Part model, mm, in its own coordinate system. Coordinates: 2 decimals unless noted, no trailing zeros. Loops run counter-clockwise (first coordinate to the right, second up) from the corner with the lowest first, then second, coordinate; pieces in that order, holes last. Notation, with made-up numbers: M 24,79 L 68,79 A23 ccw 68,89 Z; hole C 66,-37.75 d8. An arc over 180 degrees is marked long. Use a Markdown table: item, result. Add a question column.
1) Band-saw the part on D-D (y = 5). List the corners of the cut face in (x, z), plus the area to 3 significant figures.
2) Band-saw the part on A-A (x = 91). List the corners of the cut face in (y, z), plus the area to 3 significant figures.
3) Wall check: probe 1 along X at (y, z) = (35, 1.2); probe 2 along Y at (x, z) = (83, 0.8); probe 3 along X at (y, z) = (117, 1.55). Give the ranges that are in metal, low to high. Write a range as from..to.
4) Band-saw the part on B-B (y = 31). List the corners of the cut face in (x, z), plus the area to 3 significant figures.
5) Band-saw the part on C-C (x = 40). List the corners of the cut face in (y, z).
6) Pin check, flat tips, straight feed: pin 1 Ø0.8 at (x, z) = (101, 2.5) entering from +Y; pin 2 Ø0.8 at (y, z) = (28.5, 2.5) entering from -X; pin 3 Ø3.5 at (x, y) = (40, 117) entering from +Z. Stop position of each tip, or through.
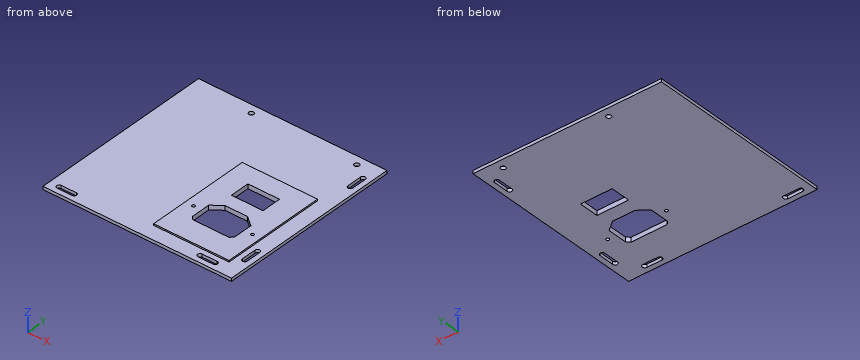
from build123d import *

# Parameters (mm, degrees)
SKETCH_W        = 125
SKETCH_H        = 123
PAD_DEPTH       = 2
SKETCH001_W     = 50
SKETCH001_H     = 70
PAD001_DEPTH    = 3
POCKET_DEPTH    = 3.001
POCKET001_DEPTH = 3.001
SKETCH004_R     = 1.6
POCKET002_DEPTH = 3.001
SKETCH005_R     = 1.6
POCKET003_DEPTH = 3.001
POCKET004_DEPTH = 3.001
SKETCH007_R     = 1
POCKET005_DEPTH = 3.001
SKETCH008_R     = 1
POCKET006_DEPTH = 3.001
SKETCH009_W     = 21
SKETCH009_H     = 13
POCKET007_DEPTH = 3.001
POCKET008_DEPTH = 3.001
POCKET009_DEPTH = 3.001


with BuildPart() as part:
    # Sketch → Pad (new body)
    with BuildSketch(Plane.XY):
        with Locations((62.5, 61.5)):
            Rectangle(SKETCH_W, SKETCH_H)
    extrude(amount=PAD_DEPTH)

    # Sketch001 → Pad001 (join)
    with BuildSketch(Plane.XY):
        with Locations((90, 45)):
            Rectangle(SKETCH001_W, SKETCH001_H)
    extrude(amount=PAD001_DEPTH)

    # Sketch002 → Pocket (cut, through all)
    with BuildSketch(Plane.XY):
        with BuildLine():
            ThreePointArc((6.55, 6.6), (4.95, 5), (6.55, 3.4))
            Line((6.55, 3.4), (16.55, 3.4))
            ThreePointArc((16.55, 3.4), (18.15, 5), (16.55, 6.6))
            Line((6.55, 6.6), (16.55, 6.6))
        make_face()
    extrude(amount=POCKET_DEPTH, mode=Mode.SUBTRACT)

    # Sketch003 → Pocket001 (cut, through all)
    with BuildSketch(Plane.XY):
        with BuildLine():
            ThreePointArc((121.6, 26.55), (120, 28.15), (118.4, 26.55))
            Line((118.4, 26.55), (118.4, 16.55))
            ThreePointArc((118.4, 16.55), (120, 14.95), (121.6, 16.55))
            Line((121.6, 26.55), (121.6, 16.55))
        make_face()
    extrude(amount=POCKET001_DEPTH, mode=Mode.SUBTRACT)

    # Sketch004 → Pocket002 (cut, through all)
    with BuildSketch(Plane.XY):
        with Locations((110, 117)):
            Circle(SKETCH004_R)
    extrude(amount=POCKET002_DEPTH, mode=Mode.SUBTRACT)

    # Sketch005 → Pocket003 (cut, through all)
    with BuildSketch(Plane.XY):
        with Locations((40, 117)):
            Circle(SKETCH005_R)
    extrude(amount=POCKET003_DEPTH, mode=Mode.SUBTRACT)

    # Sketch006 → Pocket004 (cut, through all)
    with BuildSketch(Plane.XY):
        Polygon((76, 40.43372), (82.5, 45.5), (97.5, 45.5), (104, 40.435902), (104, 27.5), (102, 25.5), (78, 25.5), (76, 27.5), align=None)
    extrude(amount=POCKET004_DEPTH, mode=Mode.SUBTRACT)

    # Sketch007 → Pocket005 (cut, through all)
    with BuildSketch(Plane.XY):
        with Locations((70.5, 35)):
            Circle(SKETCH007_R)
    extrude(amount=POCKET005_DEPTH, mode=Mode.SUBTRACT)

    # Sketch008 → Pocket006 (cut, through all)
    with BuildSketch(Plane.XY):
        with Locations((109.5, 35)):
            Circle(SKETCH008_R)
    extrude(amount=POCKET006_DEPTH, mode=Mode.SUBTRACT)

    # Sketch009 → Pocket007 (cut, through all)
    with BuildSketch(Plane.XY):
        with Locations((89.75, 61)):
            Rectangle(SKETCH009_W, SKETCH009_H)
    extrude(amount=POCKET007_DEPTH, mode=Mode.SUBTRACT)

    # Sketch010 → Pocket008 (cut, through all)
    with BuildSketch(Plane.XY):
        with BuildLine():
            ThreePointArc((100, 6.6), (98.4, 5), (100, 3.4))
            Line((100, 3.4), (110, 3.4))
            ThreePointArc((110, 3.4), (111.6, 5), (110, 6.6))
            Line((100, 6.6), (110, 6.6))
        make_face()
    extrude(amount=POCKET008_DEPTH, mode=Mode.SUBTRACT)

    # Sketch011 → Pocket009 (cut, through all)
    with BuildSketch(Plane.XY):
        with BuildLine():
            ThreePointArc((121.6, 110), (120, 111.6), (118.4, 110))
            Line((118.4, 110), (118.4, 100))
            ThreePointArc((118.4, 100), (120, 98.4), (121.6, 100))
            Line((121.6, 110), (121.6, 100))
        make_face()
    extrude(amount=POCKET009_DEPTH, mode=Mode.SUBTRACT)


solid = part.part
Entries:
| question | item | result |
|---|---|---|
| 1 | outline | M 0,0 L 4.95,0 L 4.95,2 L 0,2 Z; M 18.15,0 L 98.4,0 L 98.4,2 L 18.15,2 Z; M 111.6,0 L 125,0 L 125,2 L 111.6,2 Z |
| 1 | area | 197 mm2 |
| 2 | outline | M 0,0 L 25.5,0 L 25.5,3 L 10,3 L 10,2 L 0,2 Z; M 45.5,0 L 54.5,0 L 54.5,3 L 45.5,3 Z; M 67.5,0 L 123,0 L 123,2 L 80,2 L 80,3 L 67.5,3 Z |
| 2 | area | 217 mm2 |
| 3 | probe 1 | 0..69.5, 71.5..76, 104..108.5, 110.5..125 |
| 3 | probe 2 | 0..25.5, 45.5..54.5, 67.5..123 |
| 3 | probe 3 | 0..38.4, 41.6..108.4, 111.6..125 |
| 4 | outline | M 0,0 L 76,0 L 76,3 L 65,3 L 65,2 L 0,2 Z; M 104,0 L 125,0 L 125,2 L 115,2 L 115,3 L 104,3 Z |
| 4 | area | 216 mm2 |
| 5 | outline | M 0,0 L 115.4,0 L 115.4,2 L 0,2 Z; M 118.6,0 L 123,0 L 123,2 L 118.6,2 Z |
| 6 | pin 1 | y = 80 |
| 6 | pin 2 | x = 65 |
| 6 | pin 3 | z = 2 |
